For this review, take the finished solid that the model builds, in its own axes (mm). Round coordinates to 2 decimals unless told otherwise and drop trailing zeros. Write each loop counter-clockwise with the first axis right and the second up, starting at its lowest first coordinate (ties: lowest second). Pieces come first, ordered by that corner, then holes. Notation, with made-up numbers: M -19.75,-30 L -2.75,-30 A23 ccw -2.75,-5 Z; hole C 68,34 d5. An arc over 180 degrees is marked long. Write each question's results on one line, items separated by ' | '. Start each with the question number.
```python
from build123d import *

# Parameters (mm, degrees)
SKETCH1_W           = 34
SKETCH1_H           = 46.5
BOSS_EXTRUDE1_DEPTH = 28.5
SKETCH2_R           = 1.45
CUT_EXTRUDE1_DEPTH  = 51.088047476


with BuildPart() as part:
    # Sketch1 → Boss-Extrude1 (new body)
    with BuildSketch(Plane.XY):
        Rectangle(SKETCH1_W, SKETCH1_H)
    extrude(amount=BOSS_EXTRUDE1_DEPTH)

    # Sketch2 → Cut-Extrude1 (cut, through all)
    with BuildSketch(Plane(origin=(17, 0, 0), x_dir=(0, 0, -1), z_dir=(1, 0, 0))):
        with Locations(Location((-25.25, 20, 0), (0, 0, 90))):
            Circle(SKETCH2_R)
        with Locations(Location((-3.25, 20, 0), (0, 0, 90))):
            Circle(SKETCH2_R)
        with Locations(Location((-3.25, -20, 0), (0, 0, 90))):
            Circle(SKETCH2_R)
        with Locations(Location((-25.25, -20, 0), (0, 0, 90))):
            Circle(SKETCH2_R)
    extrude(amount=-CUT_EXTRUDE1_DEPTH, mode=Mode.SUBTRACT)


solid = part.part
```
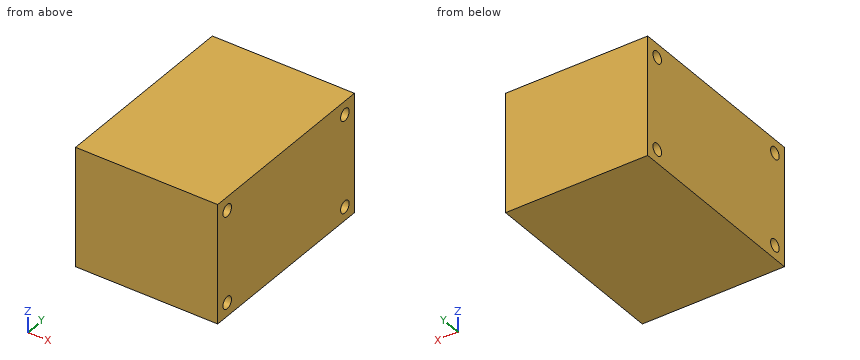
Item 1: We need section C-C on x = -3. State the section outline as (y, z) points.
Item 2: We need section A-A on y = -20. State the section outline as (x, z) points, then the cut area to 3 significant figures.
Item 3: We need section B-B on z = 3.25. State the section outline as (x, y) points.
Item 4: For probe 1 along Z at (x, y) = (7, -20); probe 2 along Y at (x, z) = (4, 26.25); probe 3 along Y at (x, z) = (-1, 25.5), list the stretches that pass through material, from the lowest coordinate up.
Item 5: Insertion check: P1, Ø1.7, axis at y = 20, z = 25.25, coming from the +X side. The pin has a flat end and moves straight along its axis. Give the tip position at first contact, or say it passes through.
Numbers:
1) outline: M -23.25,0 L 23.25,0 L 23.25,28.5 L -23.25,28.5 Z; hole C -20,3.25 d2.9; hole C -20,25.25 d2.9; hole C 20,3.25 d2.9; hole C 20,25.25 d2.9
2) outline: M -17,0 L 17,0 L 17,1.8 L -17,1.8 Z; M -17,4.7 L 17,4.7 L 17,23.8 L -17,23.8 Z; M -17,26.7 L 17,26.7 L 17,28.5 L -17,28.5 Z | area: 772 mm^2
3) outline: M -17,-23.25 L 17,-23.25 L 17,-21.45 L -17,-21.45 Z; M -17,-18.55 L 17,-18.55 L 17,18.55 L -17,18.55 Z; M -17,21.45 L 17,21.45 L 17,23.25 L -17,23.25 Z
4) probe 1: z = 0 to 1.8, 4.7 to 23.8, 26.7 to 28.5 | probe 2: y = -23.25 to -21.05, -18.95 to 18.95, 21.05 to 23.25 | probe 3: y = -23.25 to -21.43, -18.57 to 18.57, 21.43 to 23.25
5) P1: passes through
